Part model, mm, in its own coordinate system. A direction names the side the tool comes from. Round coordinates to 2 decimals unless told otherwise and drop trailing zeros. Write each loop counter-clockwise with the first axis right and the second up, starting at its lowest first coordinate (ties: lowest second). Pieces come first, ordered by that corner, then holes. Notation, with made-up numbers: M 78.25,42.25 L 108.25,42.25 A10 cw 108.25,59.25 Z; hole C 68,37 d4. An arc over 180 degrees is marked long. One line per question, with ' | ' between items. Start each with the question number.
1) Drop flat-ended pins along their axis: pin 1 Ø1 at (x, z) = (5.5, -2) entering from +Y; pin 2 Ø8 at (x, y) = (2.5, -3.5) entering from -Z; pin 3 Ø1.8 at (x, z) = (3, 4.5) entering from +Y. Give the stop position or say it passes through.
2) Mould opens along X. For faces 1 (the face through (-23, -15, 5)), 2 (the face through (13.951, -30, 1)), 3 (the face through (-4.046, -39.26, -10.736)) say: pulls with the +X half, pulls with the -X half, needs draft (parallel to the pull), parting line crosses it, or undercut.
3) Saw through at D-D (x = -24.5). List the corners of the cut face in (y, z).
4) Saw through at A-A (x = 8). List the corners of the cut face in (y, z).
5) Saw through at C-C (z = 2). List the corners of the cut face in (x, y), plus the area to 3 significant figures.
6) Tool access for faces 4 (the face through (22, -15, 5)), 5 (the face through (22, 4, 8)), 6 (the face through (26, 2, 5)), 7 (the face through (-16.049, -30, 1)): list every direction of +Z, -Z, +X, -X, +Y, -Y with a clear straight run to the whole face (end or side of a thin tool).
7) Wall check: probe 1 along X at (y, z) = (11, 7); probe 2 along Z at (x, y) = (24, 9.5); probe 3 along Y at (x, z) = (9.5, -20). Give the ranges that are in metal, low to high. Write a range as [from, to].
8) Saw through at B-B (y = -3). List the corners of the cut face in (x, z), plus the area to 3 significant figures.
```python
from build123d import *

# Parameters (mm, degrees)
ESQUISSE1_W             = 60
ESQUISSE1_H             = 30
ESQUISSE1_W_2           = 30
ESQUISSE1_H_2           = 25
BOSS_EXTRU_1_DEPTH      = 3
ESQUISSE2_W             = 30
ESQUISSE2_H             = 25
BOSS_EXTRU_2_DEPTH      = 3.5
ESQUISSE3_W             = 30
ESQUISSE3_H             = 25
BOSS_EXTRU_3_DEPTH      = 3
ESQUISSE4_W             = 30
ESQUISSE4_H             = 2.5
BOSS_EXTRU_4_DEPTH      = 22
ESQUISSE6_R             = 3
ENL_V_MAT_EXTRU_1_DEPTH = 1.5
ESQUISSE7_R             = 1.5
ENL_V_MAT_EXTRU_2_DEPTH = 6
ESQUISSE8_R             = 0.5
ENL_V_MAT_EXTRU_3_DEPTH = 10


with BuildPart() as part:
    # Esquisse1 → Boss.-Extru.1 (new body)
    with BuildSketch(Plane.XY):
        Rectangle(ESQUISSE1_W, ESQUISSE1_H)
        with Locations((-1.048951049, -27.5)):
            Rectangle(ESQUISSE1_W_2, ESQUISSE1_H_2)
    extrude(amount=BOSS_EXTRU_1_DEPTH)

    # Esquisse2 → Boss.-Extru.2 (add)
    with BuildSketch(Plane.XY.offset(3)):
        Polygon((-26, 15), (-30, 15), (-30, -15), (-26, -15), (-26, -11), align=None)
        Polygon((26, -11), (-26, -11), (-26, -15), (-16.048951049, -15), (13.951048951, -15), (26, -15), align=None)
        Polygon((26, 15), (26, -11), (26, -15), (30, -15), (30, 15), align=None)
        with Locations((-1.048951049, -27.5)):
            Rectangle(ESQUISSE2_W, ESQUISSE2_H)
    extrude(amount=BOSS_EXTRU_2_DEPTH)

    # Esquisse3 → Boss.-Extru.3 (add)
    with BuildSketch(Plane.XY.offset(6.5)):
        Polygon((-22, 15), (-30, 15), (-30, -15), (-22, -15), (-22, -8), align=None)
        Polygon((22, -8), (-22, -8), (-22, -15), (-16.048951049, -15), (13.951048951, -15), (22, -15), align=None)
        Polygon((22, 15), (22, -8), (22, -15), (30, -15), (30, 15), align=None)
        with Locations((-1.048951049, -27.5)):
            Rectangle(ESQUISSE3_W, ESQUISSE3_H)
    extrude(amount=BOSS_EXTRU_3_DEPTH)

    # Esquisse4 → Boss.-Extru.4 (add)
    with BuildSketch(Plane(origin=(0, 0, 0), x_dir=(-1, 0, 0), z_dir=(0, 0, -1))):
        with Locations((1.048951049, -38.75)):
            Rectangle(ESQUISSE4_W, ESQUISSE4_H)
    extrude(amount=BOSS_EXTRU_4_DEPTH)

    # Esquisse6 → Enlèv. mat.-Extru.1 (cut)
    with BuildSketch(Plane.XZ.offset(40)):
        with Locations((-1.048951049, -10.86835965)):
            Circle(ESQUISSE6_R)
    extrude(amount=-ENL_V_MAT_EXTRU_1_DEPTH, mode=Mode.SUBTRACT)

    # Esquisse7 → Enlèv. mat.-Extru.2 (cut)
    with BuildSketch(Plane.XZ.offset(38.5)):
        with Locations((-1.048951049, -10.86835965)):
            Circle(ESQUISSE7_R)
    extrude(amount=-ENL_V_MAT_EXTRU_2_DEPTH, mode=Mode.SUBTRACT)

    # Esquisse8 → Enlèv. mat.-Extru.3 (cut)
    with BuildSketch(Plane.XZ.offset(40)):
        with Locations((-1.048951049, -4.86835965)):
            Circle(ESQUISSE8_R)
        with Locations((-1.048951049, -16.86835965)):
            Circle(ESQUISSE8_R)
        with Locations((4.951048951, -10.86835965)):
            Circle(ESQUISSE8_R)
        with Locations((-7.048951049, -10.86835965)):
            Circle(ESQUISSE8_R)
    extrude(amount=-ENL_V_MAT_EXTRU_3_DEPTH, mode=Mode.SUBTRACT)


solid = part.part
```
Answer key:
1) pin 1: stops at y = -37.5 | pin 2: stops at z = 0 | pin 3: stops at y = -11
2) face 1: needs draft | face 2: pulls with the +X half | face 3: undercut
3) outline: M -15,0 L 15,0 L 15,3 L -11,3 L -11,6.5 L 15,6.5 L 15,9.5 L -15,9.5 Z
4) outline: M -40,-22 L -37.5,-22 L -37.5,0 L 15,0 L 15,3 L -11,3 L -11,6.5 L -8,6.5 L -8,9.5 L -40,9.5 Z
5) outline: M -30,-15 L -16.05,-15 L -16.05,-40 L 13.95,-40 L 13.95,-15 L 30,-15 L 30,15 L -30,15 Z | area: 2,550 mm2
6) face 4: +Z, -Z, +X, -Y | face 5: +Z, +Y | face 6: +Y | face 7: +Z, -Z, -X, -Y
7) probe 1: x = [-30, -22], [22, 30] | probe 2: z = [0, 3], [6.5, 9.5] | probe 3: y = [-40, -37.5]
8) outline: M -30,0 L 30,0 L 30,9.5 L 22,9.5 L 22,6.5 L 26,6.5 L 26,3 L -26,3 L -26,6.5 L -22,6.5 L -22,9.5 L -30,9.5 Z | area: 256 mm2
